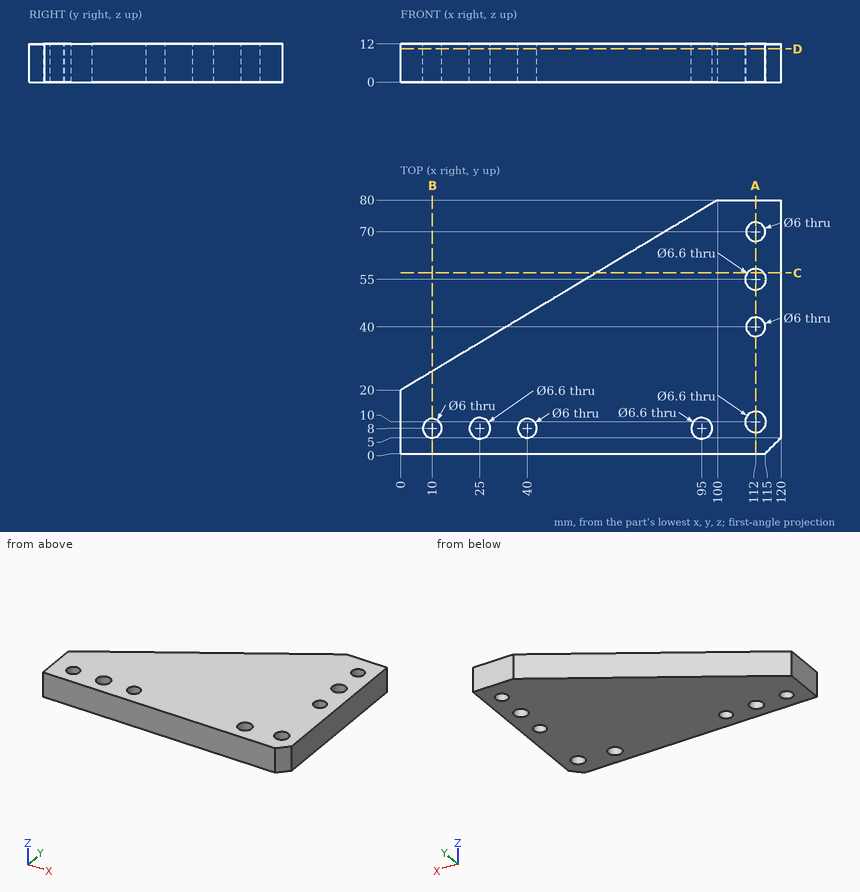
Source: three-view drawing plus pictorial views. Frame: mm from the lowest corner of the part. Round coordinates to 2 decimals unless told otherwise and drop trailing zeros. Write each loop counter-clockwise with the first axis right and the second up, starting at its lowest first coordinate (ties: lowest second). Pieces come first, ordered by that corner, then holes. Notation, with made-up numbers: M 9.5,22.5 L 67.5,22.5 A22 ccw 67.5,42.5 Z; hole C 86,81.5 d6. An arc over 180 degrees is marked long. Write item = value, one per line.
Item 1: Section query A-A on x = 112. Return loops of the section in (y, z), then the cut area to 3 significant figures.
Findings:
outline = M 0,0 L 6.7,0 L 6.7,12 L 0,12 Z; M 13.3,0 L 37,0 L 37,12 L 13.3,12 Z; M 43,0 L 51.7,0 L 51.7,12 L 43,12 Z; M 58.3,0 L 67,0 L 67,12 L 58.3,12 Z; M 73,0 L 80,0 L 80,12 L 73,12 Z
area = 658 mm^2
Item 2: Section query D-D on z = 10.5. State how many separate pieces and enclosed holes the cut face has, then the cut area to 3 significant figures.
Findings:
separate_pieces = 1
enclosed_holes = 8
area = 6,340 mm^2
Item 3: Section query B-B on x = 10. Return loops of the section in (y, z).
Findings:
outline = M 0,0 L 5,0 L 5,12 L 0,12 Z; M 11,0 L 26,0 L 26,12 L 11,12 Z
Item 4: Material intervals for line 1 along Y through (x, z) = (93, 3.5); line 2 along Y through (x, z) = (40, 5.5); line 3 along Y through (x, z) = (76.5, 7.75), sorted ascending. Write a range as [from, to].
Findings:
line_1 = [0, 5.38], [10.62, 75.8]
line_2 = [0, 5], [11, 44]
line_3 = [0, 65.9]
Item 5: Section query C-C on y = 57. Return loops of the section in (x, z).
Findings:
outline = M 61.67,0 L 109.38,0 L 109.38,12 L 61.67,12 Z; M 114.62,0 L 120,0 L 120,12 L 114.62,12 Z
Item 6: Pin query (flat end, axial travel): P1, Ø1.5, axis at y = 61, z = 1.5, coming from the -X side; P2, Ø4, axis at x = 25, y = 8, coming from the +Z side; P3, Ø1, axis at y = 59, z = 5.5, coming from the -X side; P4, Ø1, axis at x = 32, z = 1.5, coming from the +Y side. Return the tip coordinate at first contact, or that it passes through.
Findings:
P1 = 67.08
P2 = through
P3 = 64.17
P4 = 39.5
